Geometry check sheet. Reference: drawing and pictorial views, mm from the part's lowest x, y, z. A direction names the side the tool comes from. Round coordinates to 2 decimals unless told otherwise and drop trailing zeros. Order: outer loops, then holes, each group sorted by start corner. A loop starts at its lowest first (then second) coordinate and runs counter-clockwise, first axis right, second up.
(1) Mould release check, pull along X, two halves, no side actions. Record for the marked faces 1, 2 and 3: released by +X, released by -X, zero draft, split by the parting line, or undercut.
(2) Thickness scan on probe 1 along X at (y, z) = (35.5, 15.5); probe 2 along X at (y, z) = (27, 17); probe 3 along X at (y, z) = (12, 13). Record the ranges inside material, lowest first.
(3) Tool access check on the marked faces 4, 5 and 6. Record the directions out of +Z, -Z, +X, -X, +Y, -Y that give a thin tool (end or side, any length) a straight path to the whole face; none if there is none.
(4) Depth check by flat-ended pin: pin 1 (10.5 mm diameter, centred on y = 6, z = 23.5, fed in from -X); pin 2 (6.5 mm diameter, centred on y = 8, z = 17, fed in from +X); pin 3 (20.5 mm diameter, centred on y = 30, z = 14.5, fed in from +X); pin 4 (10 mm diameter, centred on x = 25.39, y = 26.85, fed in from -Z). Enter the tip coordinate at first touch or a pass-through.
(5) Sectioned sample at A-A, the plane y = 26. Enter the section's corners in (x, z) (1 decimal).
(6) Sectioned sample at C-C, the plane x = 47. Enter the section's corners in (y, z) (1 decimal), and give its area (3 significant figures).
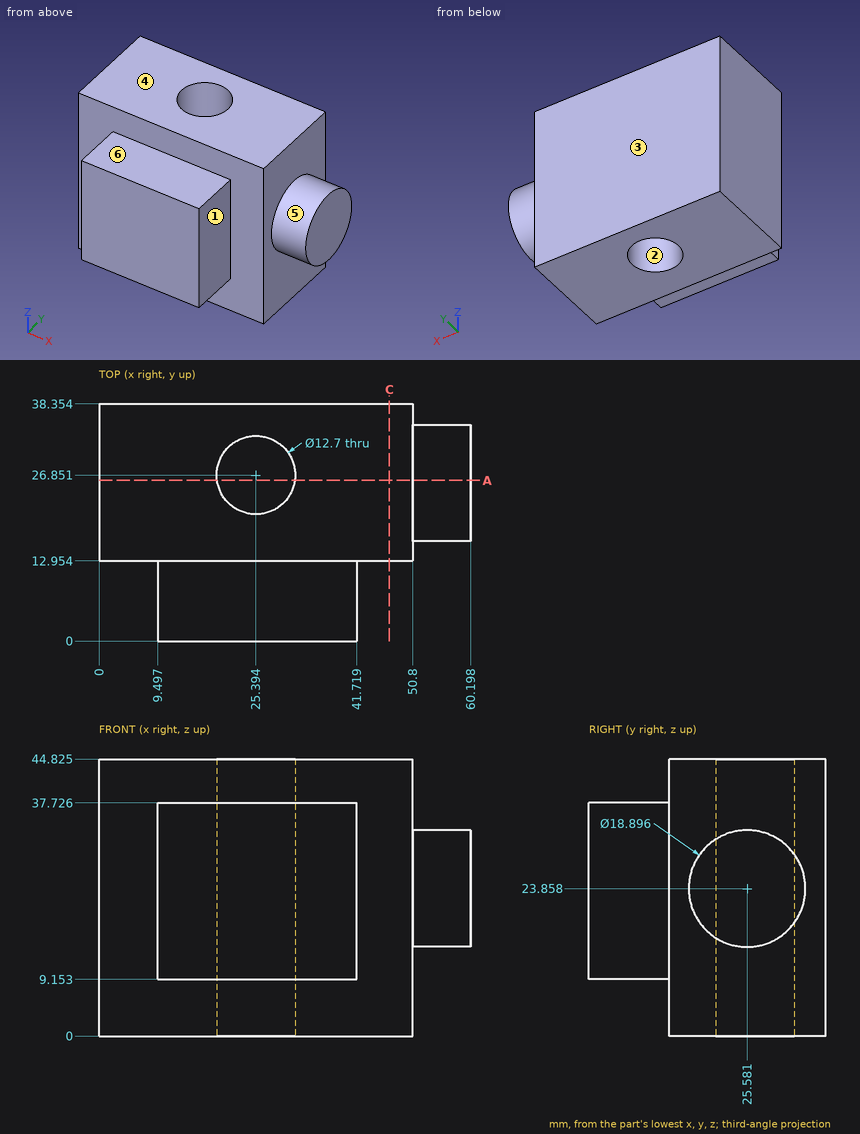
Derived:
1. face 1: released by +X
1. face 2: undercut
1. face 3: zero draft
2. probe 1: x = 0 to 50.8
2. probe 2: x = 0 to 19.05, 31.74 to 60.2
2. probe 3: x = 9.5 to 41.72
3. face 4: +Z, +X, -X, +Y, -Y
3. face 5: +X
3. face 6: +Z, +X, -X, -Y
4. pin 1: stops at x = 9.5
4. pin 2: stops at x = 41.72
4. pin 3: stops at x = 60.2
4. pin 4: passes through
5. outline: (0, 0) - (19.1, 0) - (19.1, 44.8) - (0, 44.8) - close; (31.7, 0) - (50.8, 0) - (50.8, 14.4) - (60.2, 14.4) - (60.2, 33.3) - (50.8, 33.3) - (50.8, 44.8) - (31.7, 44.8) - close
6. outline: (13, 0) - (38.4, 0) - (38.4, 44.8) - (13, 44.8) - close
6. area: 1,140 mm2
